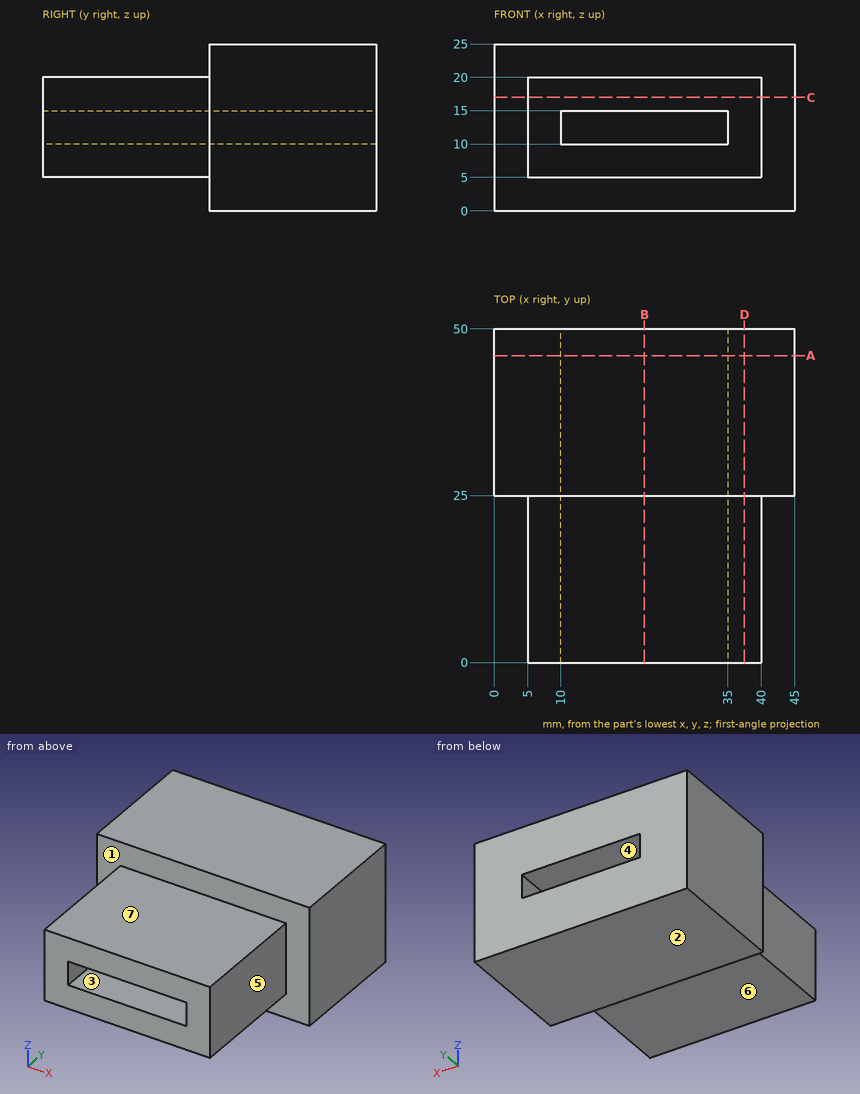
Verification items for this drawing (mm, ordinates from the low corner). A direction names the side the tool comes from. Coordinates: 2 decimals unless noted, no trailing zeros. Loops run counter-clockwise (first coordinate to the right, second up) from the corner with the lowest first, then second, coordinate; pieces in that order, holes last. Notation, with made-up numbers: (-18, 28.25) -> (8, 28.25) arc R11 ccw to (8, 44.25) -> close; hole circle Ø4 at (-40, 82.25). An arc over 180 degrees is marked (long way). Put each result on its own line as item: value.
1. Gauge pin test, flat ends, axial feed: P1, Ø3, axis at x = 28, y = 33.5, coming from the -Z side; P2, Ø4, axis at x = 25.5, y = 5.5, coming from the +Z side; P3, Ø5, axis at x = 15, y = 14.5, coming from the -Z side; P4, Ø1.5, axis at y = 23.5, z = 12.5, coming from the -X side. Record the tip position at first contact, or that the pin passes through.
Result set:
P1: stops at z = 0
P2: stops at z = 20
P3: stops at z = 5
P4: stops at x = 5
2. Thickness scan on line 1 (X direction, y = 45, z = 12.5); line 2 (Z direction, x = 24.5, y = 38.5); line 3 (Z direction, x = 22.5, y = 15.5). Record the ranges inside material, lowest first.
Result set:
line 1: x = 0 to 10, 35 to 45
line 2: z = 0 to 10, 15 to 25
line 3: z = 5 to 10, 15 to 20
3. Tool access check on the marked faces 4, 5, 6 and 7. Record the directions out of +Z, -Z, +X, -X, +Y, -Y that give a thin tool (end or side, any length) a straight path to the whole face; none if there is none.
Result set:
face 4: +Y, -Y
face 5: +Z, -Z, +X, -Y
face 6: -Z, +X, -X, -Y
face 7: +Z, +X, -X, -Y
4. Section check A-A, the plane y = 46. Record the boundary of the cut face in (x, z), then the cut area to 3 significant figures.
Result set:
outline: (0, 0) -> (45, 0) -> (45, 25) -> (0, 25) -> close; hole (10, 10) -> (35, 10) -> (35, 15) -> (10, 15) -> close
area: 1,000 mm^2
5. Section check B-B, the plane x = 22.5. Record the boundary of the cut face in (y, z).
Result set:
outline: (0, 5) -> (25, 5) -> (25, 0) -> (50, 0) -> (50, 10) -> (0, 10) -> close; (0, 15) -> (50, 15) -> (50, 25) -> (25, 25) -> (25, 20) -> (0, 20) -> close
6. Mould release check, pull along Z, two halves, no side actions. Record for the marked faces 1, 2 and 3: pulls with the +Z half, pulls with the -Z half, needs draft (parallel to the pull), parting line crosses it, or undercut.
Result set:
face 1: needs draft
face 2: pulls with the -Z half
face 3: undercut
7. Section check C-C, the plane z = 17. Record the boundary of the cut face in (x, y), then the cut area to 3 significant figures.
Result set:
outline: (0, 25) -> (5, 25) -> (5, 0) -> (40, 0) -> (40, 25) -> (45, 25) -> (45, 50) -> (0, 50) -> close
area: 2,000 mm^2
8. Section check D-D, the plane x = 37.5. Record the boundary of the cut face in (y, z), then the cut area to 3 significant figures.
Result set:
outline: (0, 5) -> (25, 5) -> (25, 0) -> (50, 0) -> (50, 25) -> (25, 25) -> (25, 20) -> (0, 20) -> close
area: 1,000 mm^2
